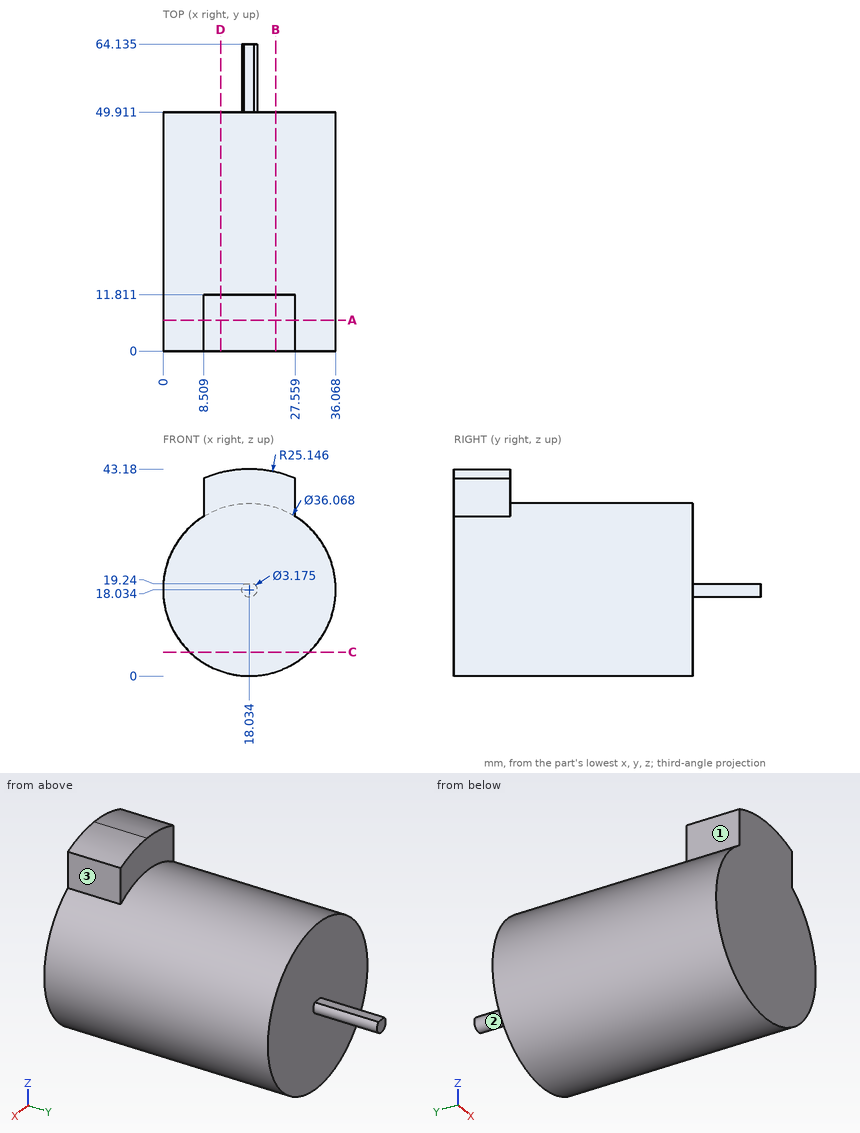
Here's the drawing with two shaded views (mm, measured from the low corner). I have some questions. A direction names the side the tool comes from. Round coordinates to 2 decimals unless told otherwise and drop trailing zeros. Order: outer loops, then holes, each group sorted by start corner. A loop starts at its lowest first (then second) coordinate and runs counter-clockwise, first axis right, second up. Notation, with made-up numbers: (-11.5, 15.5) -> (43.5, 15.5) arc R25 cw to (43.5, 47.5) -> close; hole circle Ø10 at (39, 68.25). An arc over 180 degrees is marked (long way). Return JSON: item names as keys, results as strings.
Q1. For pin 1 Ø12 at (x, z) = (10, 27.5) entering from +Y; pin 2 Ø1.7 at (x, y) = (17.5, 55.5) entering from +Z; pin 3 Ø3 at (x, y) = (5.5, 22) entering from -Z, each with a flat end and sliding along its axis, tell me the tip position at first contact or that it passes through.
Filled sheet:
{"pin 1": "stops at y = 49.91", "pin 2": "stops at z = 19.24", "pin 3": "stops at z = 3.77"}
Q2. If we section it at A-A on y = 6.5: List the corners of the cut face in (x, z) for me (1 decimal), plus the area to 3 significant figures.
Filled sheet:
{"outline": "(8.5, 33.3) arc R18 ccw (long way) to (27.6, 33.3) -> (27.6, 41.3) arc R25.1 ccw to (8.5, 41.3) -> close", "area": "1,160 mm^2"}
Q3. I need wall thicknesses on line 1 along Y through (x, z) = (9, 10); line 2 along Y through (x, z) = (22, 39); line 3 along Z through (x, y) = (33, 25) (1 decimal). Which ranges of each line are inside material? Lowest first, please. Write a range as from..to.
Filled sheet:
{"line 1": "y = 0..49.91", "line 2": "y = 0..11.81", "line 3": "z = 8..28.1"}
Q4. If we section it at B-B on x = 23.5: List the corners of the cut face in (y, z) for me, plus the area to 3 significant figures.
Filled sheet:
{"outline": "(0, 0.85) -> (49.91, 0.85) -> (49.91, 35.22) -> (11.81, 35.22) -> (11.81, 42.58) -> (0, 42.58) -> close", "area": "1,800 mm^2"}
Q5. If we section it at C-C on z = 5: List the corners of the cut face in (x, y) for me.
Filled sheet:
{"outline": "(5.57, 0) -> (30.5, 0) -> (30.5, 49.91) -> (5.57, 49.91) -> close"}
Q6. Which directions (+Z, -Z, +X, -X, +Y, -Y) give clear straight access to the entire face, cutting with the end or side of a thin tool? Please do the marked faces 1, 2 and 3.
Filled sheet:
{"face 1": "+Z, -X, +Y, -Y", "face 2": "+Y", "face 3": "+Z, +X, +Y, -Y"}
Q7. If we section it at D-D on x = 12: List the corners of the cut face in (y, z) for me (1 decimal), plus the area to 3 significant figures.
Filled sheet:
{"outline": "(0, 1) -> (49.9, 1) -> (49.9, 35) -> (11.8, 35) -> (11.8, 42.4) -> (0, 42.4) -> close", "area": "1,780 mm^2"}
